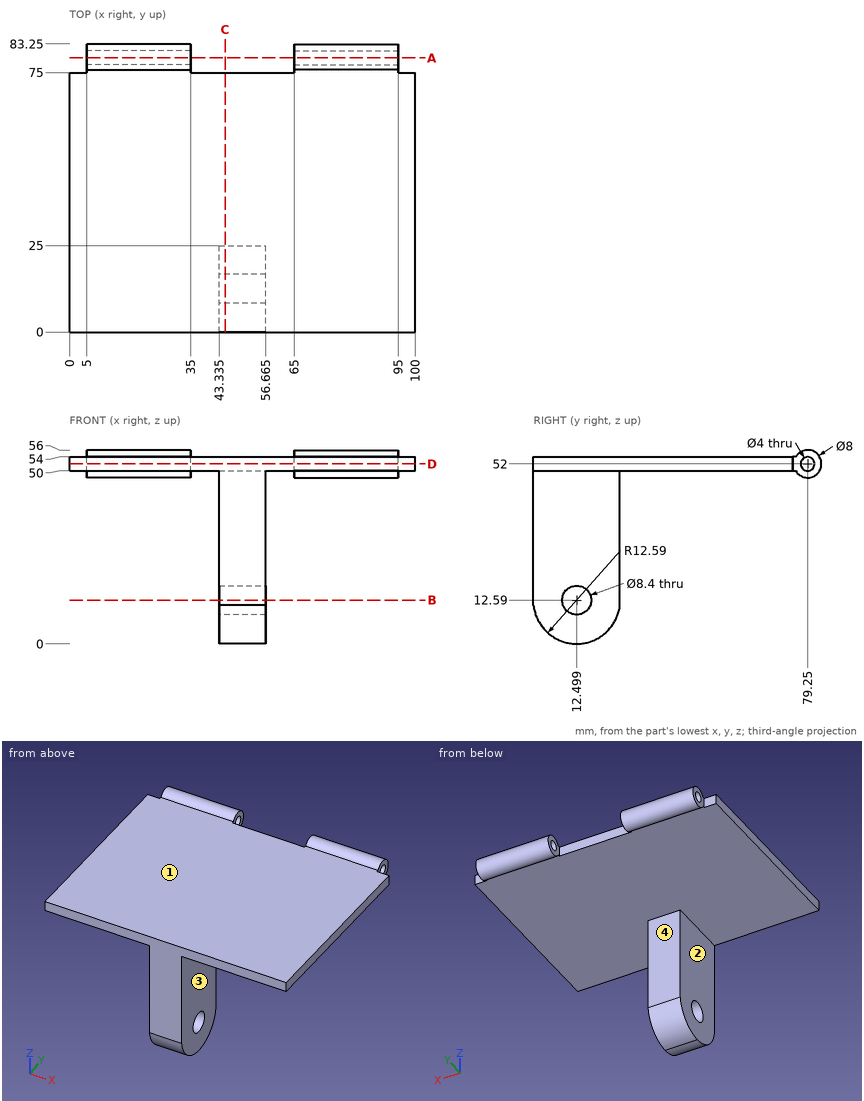
Part print with two shaded views. Sizes in mm from the minimum x, y, z corner. A direction names the side the tool comes from. Round coordinates to 2 decimals unless told otherwise and drop trailing zeros. Write each loop counter-clockwise with the first axis right and the second up, starting at its lowest first coordinate (ties: lowest second). Pieces come first, ordered by that corner, then holes. Notation, with made-up numbers: (66, 27) -> (118, 27) arc R9 cw to (118, 35) -> close; hole circle Ø7 at (-26, -1.75). An arc over 180 degrees is marked (long way). Use one line per item in the form item = value.
Q1. Band-saw the part on A-A, the plane y = 79.25. Write the cut outline in (x, z), then the cut area to 3 significant figures.
Conclusion:
outline = (5, 48) -> (35, 48) -> (35, 50) -> (5, 50) -> close; (5, 54) -> (35, 54) -> (35, 56) -> (5, 56) -> close; (65, 48) -> (95, 48) -> (95, 50) -> (65, 50) -> close; (65, 54) -> (95, 54) -> (95, 56) -> (65, 56) -> close
area = 240 mm²
Q2. Tool access for the marked faces 1, 2, 3 and 4: list every direction of +Z, -Z, +X, -X, +Y, -Y with a clear straight run to the whole face (end or side of a thin tool).
Conclusion:
face_1 = +Z, +X, -X, -Y
face_2 = -Z, -X, +Y, -Y
face_3 = -Z, +X, +Y, -Y
face_4 = -Z, +X, -X, +Y
Q3. Drop flat-ended pins along their axis: P1, Ø1, axis at x = 15, y = 61.5, coming from the +Z side; P2, Ø4, axis at y = 78, z = 54, coming from the -X side; P3, Ø4, axis at x = 27.5, y = 64.5, coming from the -Z side. Give the stop position or say it passes through.
Conclusion:
P1 = 54
P2 = 5
P3 = 50
Q4. Band-saw the part on B-B, the plane z = 12.59. Write the cut outline in (x, y) (1 decimal), then the cut area to 3 significant figures.
Conclusion:
outline = (43.3, 0) -> (56.7, 0) -> (56.7, 8.3) -> (43.3, 8.3) -> close; (43.3, 16.7) -> (56.7, 16.7) -> (56.7, 25) -> (43.3, 25) -> close
area = 221 mm²
Q5. Band-saw the part on C-C, the plane x = 45. Write the cut outline in (y, z), then the cut area to 3 significant figures.
Conclusion:
outline = (0, 11.08) arc R12.59 ccw to (25, 11.09) -> (25, 50) -> (75, 50) -> (75, 54) -> (0, 54) -> close; hole circle Ø8.4 at (12.5, 12.59)
area = 1,430 mm²
Q6. Drill centre lines: L1, parallel to Y at x = 47, z = 12.59; L2, parallel to Y at x = 21, z = 52; L3, parallel to Z at x = 72, y = 9.5. Where is each one in solid material? Low to high.
Conclusion:
L1 = 0 to 8.3, 16.7 to 25
L2 = 0 to 77.25, 81.25 to 83.25
L3 = 50 to 54
Q7. Band-saw the part on D-D, the plane z = 52. Write the cut outline in (x, y).
Conclusion:
outline = (0, 0) -> (100, 0) -> (100, 75) -> (95, 75) -> (95, 77.25) -> (65, 77.25) -> (65, 75) -> (35, 75) -> (35, 77.25) -> (5, 77.25) -> (5, 75) -> (0, 75) -> close; (5, 81.25) -> (35, 81.25) -> (35, 83.25) -> (5, 83.25) -> close; (65, 81.25) -> (95, 81.25) -> (95, 83.25) -> (65, 83.25) -> close
